Can you work these out from the drawing? Everything is in mm from the part's minimum corner. A direction names the side the tool comes from. Round coordinates to 2 decimals unless told otherwise and drop trailing zeros. Write each loop counter-clockwise with the first axis right and the second up, starting at its lowest first coordinate (ties: lowest second). Pieces come first, ordered by that corner, then holes. Notation, with made-up numbers: (-31, -38.5) -> (17, -38.5) arc R23 ccw to (17, -13.5) -> close; hole circle Ø1 at (83, 17). An arc over 180 degrees is marked (long way). Answer as CSV lines item,"result".
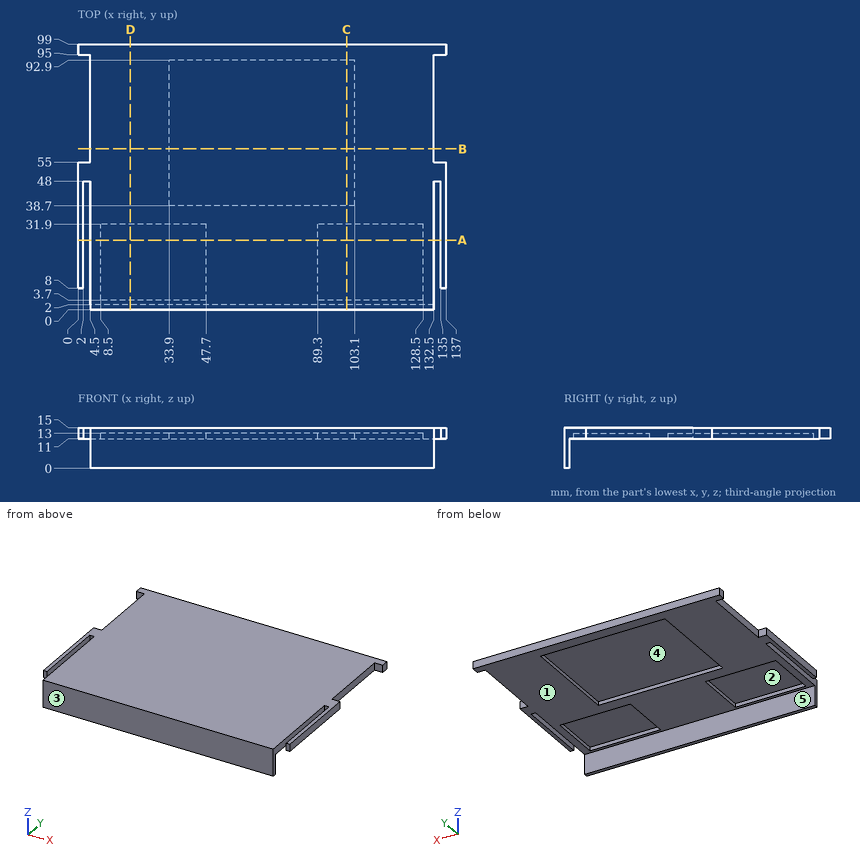
Item 1: Suppose I cut it at A-A, the plane y = 26. List the corners of the cut face in (x, z) for me, then the cut area to 3 significant figures.
Results found:
outline,"(0, 11) -> (2, 11) -> (2, 15) -> (0, 15) -> close; (4.5, 11) -> (8.5, 11) -> (8.5, 13) -> (47.7, 13) -> (47.7, 11) -> (89.3, 11) -> (89.3, 13) -> (128.5, 13) -> (128.5, 11) -> (132.5, 11) -> (132.5, 15) -> (4.5, 15) -> close; (135, 11) -> (137, 11) -> (137, 15) -> (135, 15) -> close"
area,"371 mm²"
Item 2: Suppose I cut it at D-D, the plane x = 19.5. List the corners of the cut face in (y, z) for me, then the cut area to 3 significant figures.
Results found:
outline,"(0, 0) -> (2, 0) -> (2, 11) -> (3.7, 11) -> (3.7, 13) -> (31.9, 13) -> (31.9, 11) -> (99, 11) -> (99, 15) -> (0, 15) -> close"
area,"362 mm²"
Item 3: If we mould it in two halves opening along X, with no side actions, what happens to the marked faces 4 and 5? For each: pulls with the +X half, pulls with the -X half, needs draft (parallel to the pull), parting line crosses it, or undercut.
Results found:
face 4,"undercut"
face 5,"needs draft"
Item 4: For the marked faces 1, 2 and 3, which set-ups out of +Z, -Z, +X, -X, +Y, -Y let a thin tool reach every point of the face, with its end or its side?
Results found:
face 1,"-Z, +X, -X, +Y"
face 2,"-Z"
face 3,"+Z, -Z, +X, -X, -Y"
Item 5: Suppose I cut it at B-B, the plane y = 60. List the corners of the cut face in (x, z) for me.
Results found:
outline,"(4.5, 11) -> (33.9, 11) -> (33.9, 13) -> (103.1, 13) -> (103.1, 11) -> (132.5, 11) -> (132.5, 15) -> (4.5, 15) -> close"
Item 6: Suppose I cut it at C-C, the plane x = 100. List the corners of the cut face in (y, z) for me, then the cut area to 3 significant figures.
Results found:
outline,"(0, 0) -> (2, 0) -> (2, 11) -> (3.7, 11) -> (3.7, 13) -> (31.9, 13) -> (31.9, 11) -> (38.7, 11) -> (38.7, 13) -> (92.9, 13) -> (92.9, 11) -> (99, 11) -> (99, 15) -> (0, 15) -> close"
area,"253 mm²"
Item 7: Will these pins go through, and if not, where does the flat tip stop? pin 1 (2 mm diameter, centred on y = 78, z = 13, fed in from +X); pin 2 (2 mm diameter, centred on x = 136, z = 12, fed in from -Y).
Results found:
pin 1,"stops at x = 132.5"
pin 2,"stops at y = 8"
Item 8: I need wall thicknesses on L1, parallel to X at y = 40, z = 12.75; L2, parallel to Y at x = 125, z = 4; L3, parallel to Z at x = 122, y = 64.5. Which ranges of each line are inside material? Lowest first, please.
Results found:
L1,"x = 0 to 2, 4.5 to 33.9, 103.1 to 132.5, 135 to 137"
L2,"y = 0 to 2"
L3,"z = 11 to 15"
